from build123d import *

# Parameters (mm, degrees)
SKETCH_1_R               = 21
EXTRUDE_1_DEPTH          = 3.8
SKETCH_2_R               = 17.75
EXTRUDE_2_DEPTH          = 6.2
SKETCH_3_R               = 2.1
SKETCH_3_R_2             = 8.75
CUT_EXTRUDE_1_DEPTH      = 32.336879232
CUT_EXTRUDE_2_REACH      = 50.491
CUT_EXTRUDE_2_END_RADIUS = 8.75
SKETCH_5_R               = 1.5
PATTERN_CIRCULAR_1_COUNT = 4
CUT_EXTRUDE_3_DEPTH      = 6.2


with BuildPart() as part:
    # ｽｹｯﾁ1 → ﾎﾞｽ - 押し出し1 (new body)
    with BuildSketch(Plane.XY):
        with Locations(Location((0, 0, 0), (0, 0, 180))):
            Circle(SKETCH_1_R)
    extrude(amount=EXTRUDE_1_DEPTH)

    # ｽｹｯﾁ2 → ﾎﾞｽ - 押し出し2 (add)
    with BuildSketch(Plane.XY.offset(3.8)):
        with Locations(Location((0, 0, 0), (0, 0, 180))):
            Circle(SKETCH_2_R)
    extrude(amount=EXTRUDE_2_DEPTH)

    # ｽｹｯﾁ3 → ｶｯﾄ - 押し出し1 (cut, through all)
    with BuildSketch(Plane.XY.offset(10)):
        with Locations((-14.5, 0)):
            Circle(SKETCH_3_R)
        with Locations(Location((14.5, 0, 0), (0, 0, 180))):
            Circle(SKETCH_3_R)
        Circle(SKETCH_3_R_2)
    extrude(amount=-CUT_EXTRUDE_1_DEPTH, mode=Mode.SUBTRACT)

    # ｶｯﾄ - 押し出し2: up to this cylinder (the profile starts outside it)
    cut_extrude_2_end = Plane(origin=(0, 0, 7.5), z_dir=(0, 0, 1)) * Cylinder(CUT_EXTRUDE_2_END_RADIUS, 119.482, mode=Mode.PRIVATE)
    # ｽｹｯﾁ5 → ｶｯﾄ - 押し出し2 (cut, up to the surface)
    with BuildSketch(Plane(origin=(12.551145366, 12.551145366, 0), x_dir=(0.7071067811865489, -0.7071067811865461, 0), z_dir=(0.7071067811865461, 0.7071067811865489, 0)), mode=Mode.PRIVATE) as cut_extrude_2_sk1:
        with Locations(Location((0, -7.5, 0), (0, 0, 180))):
            Circle(SKETCH_5_R)
    cut_extrude_2_tool1 = extrude(cut_extrude_2_sk1.sketch, amount=-CUT_EXTRUDE_2_REACH, mode=Mode.PRIVATE) - cut_extrude_2_end
    cut_extrude_2 = cut_extrude_2_tool1.solids().sort_by_distance((12.551145, 12.551145, 7.5))[0]
    add(cut_extrude_2, mode=Mode.SUBTRACT)

    # 円形ﾊﾟﾀｰﾝ1: ｶｯﾄ - 押し出し2 ×4 about axis
    pattern_circular_1_axis = Axis((0, 0, 10), (0, 0, -1))
    for i in range(1, PATTERN_CIRCULAR_1_COUNT):
        add(cut_extrude_2.rotate(pattern_circular_1_axis, i * 360 / PATTERN_CIRCULAR_1_COUNT), mode=Mode.SUBTRACT)

    # ｽｹｯﾁ6 → ｶｯﾄ - 押し出し3 (cut)
    with BuildSketch(Plane.XY.offset(10)):
        with BuildLine():
            Line((-14.5, -3.5), (-17.75, -3.5))
            ThreePointArc((-17.75, -3.5), (-21.25, 0), (-17.75, 3.5))
            Line((-17.75, 3.5), (-14.5, 3.5))
            ThreePointArc((-14.5, 3.5), (-11, 0), (-14.5, -3.5))
        make_face()
        with BuildLine():
            Line((14.5, -3.5), (17.75, -3.5))
            ThreePointArc((17.75, -3.5), (21.25, 0), (17.75, 3.5))
            Line((17.75, 3.5), (14.5, 3.5))
            ThreePointArc((14.5, 3.5), (11, 0), (14.5, -3.5))
        make_face()
    extrude(amount=-CUT_EXTRUDE_3_DEPTH, mode=Mode.SUBTRACT)


solid = part.part
CAD build for the part. Positions are in the model's coordinates, mm. A direction names the side the tool comes from. Coordinates: 2 decimals unless noted, no trailing zeros. Write each loop counter-clockwise with the first axis right and the second up, starting at its lowest first coordinate (ties: lowest second). Pieces come first, ordered by that corner, then holes. Notation, with made-up numbers: (-39.75, -36.5) - (15.25, -36.5) arc R24 ccw to (15.25, 2.5) - close; hole circle Ø11 at (11, 52.5). An arc over 180 degrees is marked (long way). Use a Markdown table: item, result. Add a question column.
Item 1: Drill centre lines: L1, parallel to X at y = -11.5, z = 8.5; L2, parallel to X at y = -10, z = 8 (3 decimals); L3, parallel to Z at x = 18, y = -2. Where is each one in solid material? Low to high. Write a range as from..to.
Item 2: Band-saw the part on B-B, the plane y = 0. Give the cut face in (x, z).
Item 3: Band-saw the part on C-C, the plane x = 4.5. Give the cut face in (y, z).
Item 4: Flat gauge pins, fed straight in: pin 1 (3 mm diameter, centred on x = -8, z = 3.5, fed in from +Y); pin 2 (1.5 mm diameter, centred on x = 16, z = 6.5, fed in from -Y); pin 3 (3 mm diameter, centred on y = 4.5, z = 8, fed in from -X). Where does each tip first touch, or does it go through?
Item 5: Band-saw the part on A-A, the plane x = 0. Give the cut face in (y, z).
Item 6: 3-axis set-ups, long thin cutter, end or side, ignore diameter. For faces 4 (the face through (16, -3.5, 7)), 5 (the face through (-0.341, -17.747, 6.857)), 6 (the face through (0.341, 17.747, 6.857)): which of +Z, -Z, +X, -X, +Y, -Y reach the whole face in a straight line?
Item 7: Mould opens along X. For faces 1 (the face through (-9.86, 8.88, 6.17)), 2 (the face through (-16, -3.5, 7)), 3 (the face through (-20.03, -6.31, 1.87)) say: pulls with the +X half, pulls with the -X half, needs draft (parallel to the pull), parting line crosses it, or undercut.
Numbers:
| question | item | result |
|---|---|---|
| 1 | L1 | -13.52..-13.08, -9.92..9.92, 13.08..13.52 |
| 1 | L2 | -14.665..-12, -8..8, 12..14.665 |
| 1 | L3 | 0..3.8 |
| 2 | outline | (-21, 0) - (-16.6, 0) - (-16.6, 3.8) - (-21, 3.8) - close; (-12.4, 0) - (-8.75, 0) - (-8.75, 10) - (-11, 10) - (-11, 3.8) - (-12.4, 3.8) - close; (8.75, 0) - (12.4, 0) - (12.4, 3.8) - (11, 3.8) - (11, 10) - (8.75, 10) - close; (16.6, 0) - (21, 0) - (21, 3.8) - (16.6, 3.8) - close |
| 3 | outline | (-20.51, 0) - (-7.5, 0) - (-7.5, 10) - (-17.17, 10) - (-17.17, 3.8) - (-20.51, 3.8) - close; (7.5, 0) - (20.51, 0) - (20.51, 3.8) - (17.17, 3.8) - (17.17, 10) - (7.5, 10) - close |
| 4 | pin 1 | y = 19.97 |
| 4 | pin 2 | y = -9.08 |
| 4 | pin 3 | x = -17.4 |
| 5 | outline | (-21, 0) - (-8.75, 0) - (-8.75, 10) - (-17.75, 10) - (-17.75, 3.8) - (-21, 3.8) - close; (8.75, 0) - (21, 0) - (21, 3.8) - (17.75, 3.8) - (17.75, 10) - (8.75, 10) - close |
| 6 | face 4 | +Z, +X |
| 6 | face 5 | +Z, -Y |
| 6 | face 6 | +Z, +Y |
| 7 | face 1 | undercut |
| 7 | face 2 | needs draft |
| 7 | face 3 | parting line crosses it |
